from build123d import *

# Parameters (mm, degrees)
SKETCH1_W           = 101.6
SKETCH1_H           = 60.325
BOSS_EXTRUDE1_DEPTH = 6.35
FILLET1_R           = 3.175
SKETCH2_R           = 0.635
BOSS_EXTRUDE2_DEPTH = 6.35


with BuildPart() as part:
    # Sketch1 → Boss-Extrude1 (new body)
    with BuildSketch(Plane.XY):
        Rectangle(SKETCH1_W, SKETCH1_H)
    extrude(amount=BOSS_EXTRUDE1_DEPTH)

    # Fillet1
    fillet1_edges = [part.edges().sort_by_distance(p)[0] for p in [
        (0, 30.1625, 6.35),
        (0, 30.1625, 0),
        (0, -30.1625, 6.35),
        (0, -30.1625, 0),
    ]]
    fillet(fillet1_edges, radius=FILLET1_R - 0.0001)  # a hair under: the kernel refuses the full size

    # Sketch2 → Boss-Extrude2 (add)
    with BuildSketch(Plane.ZY.offset(50.8)):
        with Locations(Location((3.175, 26.9875, 0), (0, 0, 180))):
            Circle(SKETCH2_R)
        with Locations(Location((3.175, -26.9875, 0), (0, 0, 180))):
            Circle(SKETCH2_R)
    extrude(amount=BOSS_EXTRUDE2_DEPTH)


solid = part.part
Can you work these out from the model? Positions are in its coordinate system, mm. Give positions to 0.01 mm unless a question says otherwise; leave off trailing zeros. Order: outer loops, then holes, each group sorted by start corner. A loop starts at its lowest first (then second) coordinate and runs counter-clockwise, first axis right, second up. Notation, with made-up numbers: M 60.25,3 L 77.25,3 A19 cw 77.25,19 Z; hole C -35.75,-37 d1. An arc over 180 degrees is marked long. Use a Markdown table: item, result. Add a question column.
Item 1: Will these pins go through, and if not, where does the flat tip stop? pin 1 (2 mm diameter, centred on y = -8, z = 1.5, fed in from -X); pin 2 (1 mm diameter, centred on x = 2.5, z = 1, fed in from +Y).
Item 2: Suppose I cut it at B-B (y = -14). List the corners of the cut face in (x, z) for me, then the cut area to 3 significant figures.
Item 3: If I drill on L1, parallel to X at y = 11, z = 3; L2, parallel to Y at x = 18.5, z = 3.5; L3, parallel to Y at x = -0.5, z = 3, over which ranges is the centre line in solid material (lowest first)? Write a range as [from, to].
Answer sheet:
| question | item | result |
|---|---|---|
| 1 | pin 1 | stops at x = -50.8 |
| 1 | pin 2 | stops at y = 29.68 |
| 2 | outline | M -50.8,0 L 50.8,0 L 50.8,6.35 L -50.8,6.35 Z |
| 2 | area | 645 mm² |
| 3 | L1 | x = [-50.8, 50.8] |
| 3 | L2 | y = [-30.15, 30.15] |
| 3 | L3 | y = [-30.16, 30.16] |
